Design review of the part built by this model. Coordinates are the model's own, in mm. A direction names the side the tool comes from. Give positions to 0.01 mm unless a question says otherwise; leave off trailing zeros. Loops run counter-clockwise (first coordinate to the right, second up) from the corner with the lowest first, then second, coordinate; pieces in that order, holes last. Notation, with made-up numbers: (20.5, -31) -> (62.5, -31) arc R14 cw to (62.5, -8) -> close; hole circle Ø3 at (-7, 73). An arc over 180 degrees is marked (long way). Use a Markdown table: item, result. Add a question column.
1. Draft analysis for pull direction Y (two halves, no side actions). For faces 1 (the cylindrical face through (29.57, 2.35, 21.95)), 2 (the cylindrical face through (-19.5, -19.6, 24.7)), 3 (the flat face through (0, -20, 1)), 4 (the flat face through (-2, -23, 22)), state which applies: pulls with the +Y half, pulls with the -Y half, needs draft (parallel to the pull), parting line crosses it, or undercut.
2. For pin 1 Ø4.5 at (x, y) = (35.35, -25.35) entering from +Z; pin 2 Ø10 at (x, z) = (6.5, 6) entering from -Y; pin 3 Ø5 at (y, z) = (3.5, 13) entering from +X; pin 4 Ø18.5 at (x, y) = (3.5, -11) entering from +Z, all flat-tipped, find the tip position at first contact; note any pin that passes through.
3. Add section C-C (y = -25.35). State the section outline as (x, z) points, and give its area (3 significant figures).
4. Add section B-B (y = -3). State the section outline as (x, z) points.
5. Add section A-A (z = 11.5). State the section outline as (x, y) points.
6. To check wall thickness, follow line 1 (Y direction, x = 35.35, z = 1.05); line 2 (X direction, y = -25.35, z = 1.4); line 3 (Z direction, x = 33, y = -19). State the ranges of each line that lie inside material, in increasing order.
7. Add section D-D (x = 35.35). State the section outline as (y, z) points.
8. For faces 5 (the flat face through (0, 31, 1)), 6 (the cylindrical face through (33.706, -24.302, 0.986)), 7 (the flat face through (0, 20, 1)), 8 (the flat face through (-31, 2, 10)), 9 (the cylindrical face through (19.8, 24.06, 24.68)), list the 3-axis set-ups (+Z, -Z, +X, -X, +Y, -Y) from which the entire face can be reached by the end or side of a thin tool; tool diameter is ignored.
```python
from build123d import *

# Parameters (mm, degrees)
PAD_DEPTH    = 33
SKETCH002_W  = 62
SKETCH002_H  = 21.45
PAD002_DEPTH = 25
FILLET_R     = 5
SKETCH003_R  = 1.6
PAD003_DEPTH = 2.5
SKETCH001_R  = 1.95
PAD001_DEPTH = 2
SKETCH004_W  = 40
SKETCH004_H  = 25
POCKET_DEPTH = 5


with BuildPart() as pad:
    # Sketch → Pad (new body, symmetric)
    with BuildSketch(Plane(origin=(0, 0, 2), x_dir=(1, 0, 0), z_dir=(0, -1, 0))):
        with BuildLine():
            ThreePointArc((-18.35, 19), (-27.85, 9.5), (-18.35, 0))
            Line((-18.35, 0), (18.35, 0))
            ThreePointArc((18.35, 0), (27.85, 9.5), (18.35, 19))
            Line((-18.35, 19), (18.35, 19))
        make_face()
    extrude(amount=PAD_DEPTH, both=True)


with BuildPart() as pad003:
    # Sketch002 → Pad002 (new body, symmetric)
    with BuildSketch(Plane.XZ.offset(-2)):
        with Locations((0, 12.725)):
            Rectangle(SKETCH002_W, SKETCH002_H)
    extrude(amount=PAD002_DEPTH, both=True)

    # Fillet
    fillet_edges = [pad003.edges().sort_by_distance(p)[0] for p in [
        (-31, 2, 23.45),
        (31, 2, 23.45),
    ]]
    fillet(fillet_edges, radius=FILLET_R)

    # Cut: cut Pad
    add(pad.part, mode=Mode.SUBTRACT)

    # Sketch003 → Pad003 (new body)
    with BuildSketch(Plane.XY.offset(23.45)):
        with Locations((-20.975, 22.975)):
            Circle(SKETCH003_R)
        with Locations((-20.975, -18.975)):
            Circle(SKETCH003_R)
        with Locations((20.975, 22.975)):
            Circle(SKETCH003_R)
        with Locations((20.975, -18.975)):
            Circle(SKETCH003_R)
    extrude(amount=PAD003_DEPTH)


with BuildPart() as fusion:
    # Sketch001 → Pad001 (new body)
    with BuildSketch(Plane(origin=(0, 0, 0), x_dir=(0, 1, 0), z_dir=(0, 0, 1))):
        with BuildLine():
            Line((-24.5, 40), (24.5, 40))
            ThreePointArc((31, 33.5), (29.096194, 38.096194), (24.5, 40))
            Line((31, 33.5), (31, -33.5))
            ThreePointArc((24.5, -40), (29.096194, -38.096194), (31, -33.5))
            Line((24.5, -40), (-24.5, -40))
            ThreePointArc((-31, -33.5), (-29.096194, -38.096194), (-24.5, -40))
            Line((-31, -33.5), (-31, 33.5))
            ThreePointArc((-24.5, 40), (-29.096194, 38.096194), (-31, 33.5))
        make_face()
        with Locations((-25.35, 35.35)):
            Circle(SKETCH001_R, mode=Mode.SUBTRACT)
        with Locations((25.35, 35.35)):
            Circle(SKETCH001_R, mode=Mode.SUBTRACT)
        with Locations((25.35, -35.35)):
            Circle(SKETCH001_R, mode=Mode.SUBTRACT)
        with Locations((-25.35, -35.35)):
            Circle(SKETCH001_R, mode=Mode.SUBTRACT)
    extrude(amount=PAD001_DEPTH)

    # Sketch004 → Pocket (cut)
    with BuildSketch(Plane.YX):
        Rectangle(SKETCH004_W, SKETCH004_H)
    extrude(amount=-POCKET_DEPTH, mode=Mode.SUBTRACT)

    # Fusion: union Pad003
    add(pad003.part)


solid = fusion.part
```
Taken from the geometry:
| question | item | result |
|---|---|---|
| 1 | face 1 | needs draft |
| 1 | face 2 | undercut |
| 1 | face 3 | undercut |
| 1 | face 4 | pulls with the -Y half |
| 2 | pin 1 | stops at z = 2 |
| 2 | pin 2 | stops at y = -31 |
| 2 | pin 3 | stops at x = 31 |
| 2 | pin 4 | stops at z = 23.45 |
| 3 | outline | (-39.94, 0) -> (-37.3, 0) -> (-37.3, 2) -> (-39.94, 2) -> close; (-33.4, 0) -> (33.4, 0) -> (33.4, 2) -> (-33.4, 2) -> close; (37.3, 0) -> (39.94, 0) -> (39.94, 2) -> (37.3, 2) -> close |
| 3 | area | 144 mm^2 |
| 4 | outline | (-40, 0) -> (-12.5, 0) -> (-12.5, 2) -> (-18.35, 2) arc R9.5 cw to (-18.35, 21) -> (18.35, 21) arc R9.5 cw to (18.35, 2) -> (12.5, 2) -> (12.5, 0) -> (40, 0) -> (40, 2) -> (31, 2) -> (31, 18.45) arc R5 ccw to (26, 23.45) -> (-26, 23.45) arc R5 ccw to (-31, 18.45) -> (-31, 2) -> (-40, 2) -> close |
| 5 | outline | (-31, -23) -> (-27.85, -23) -> (-27.85, 27) -> (-31, 27) -> close; (27.85, -23) -> (31, -23) -> (31, 27) -> (27.85, 27) -> close |
| 6 | line 1 | y = -30.73 to -27.3, -23.4 to 23.4, 27.3 to 30.73 |
| 6 | line 2 | x = -39.94 to -37.3, -33.4 to 33.4, 37.3 to 39.94 |
| 6 | line 3 | z = 0 to 2 |
| 7 | outline | (-30.73, 0) -> (-27.3, 0) -> (-27.3, 2) -> (-30.73, 2) -> close; (-23.4, 0) -> (23.4, 0) -> (23.4, 2) -> (-23.4, 2) -> close; (27.3, 0) -> (30.73, 0) -> (30.73, 2) -> (27.3, 2) -> close |
| 8 | face 5 | +Z, -Z, +X, -X, +Y |
| 8 | face 6 | +Z, -Z |
| 8 | face 7 | -Z |
| 8 | face 8 | +Z, -X, +Y, -Y |
| 8 | face 9 | +Z |
